```python
from build123d import *

# Parameters (mm, degrees)
SKETCH1_W           = 30
SKETCH1_H           = 90
BOSS_EXTRUDE1_DEPTH = 8
SKETCH2_W           = 10
SKETCH2_H           = 12
CUT_EXTRUDE1_DEPTH  = 8
SKETCH3_R           = 2.25
CUT_EXTRUDE2_DEPTH  = 55.671747731
FILLET1_R           = 2
CUT_EXTRUDE3_DEPTH  = 49.104053883
FILLET2_R           = 3
CHAMFER1_SIZE       = 1.5
FILLET3_R           = 0.5


with BuildPart() as part:
    # Sketch1 → Boss-Extrude1 (new body)
    with BuildSketch(Plane(origin=(0, 0, 0), x_dir=(1, 0, 0), z_dir=(0, 1, 0))):
        Rectangle(SKETCH1_W, SKETCH1_H)
    extrude(amount=BOSS_EXTRUDE1_DEPTH)

    # Sketch2 → Cut-Extrude1 (cut)
    with BuildSketch(Plane(origin=(0, 8, 0), x_dir=(1, 0, 0), z_dir=(0, 1, 0))):
        with Locations((0, 39)):
            Rectangle(SKETCH2_W, SKETCH2_H)
        with Locations((0, -39)):
            Rectangle(SKETCH2_W, SKETCH2_H)
    extrude(amount=-CUT_EXTRUDE1_DEPTH, mode=Mode.SUBTRACT)

    # Sketch3 → Cut-Extrude2 (cut, through all)
    with BuildSketch(Plane(origin=(15, 0, 0), x_dir=(0, 0, -1), z_dir=(1, 0, 0))):
        with Locations((-40, 4)):
            Circle(SKETCH3_R)
    cut_extrude2 = extrude(amount=-CUT_EXTRUDE2_DEPTH, mode=Mode.SUBTRACT)

    # Mirror1: Cut-Extrude2 across plane
    add(cut_extrude2.mirror(Plane.XY), mode=Mode.SUBTRACT)

    # Fillet1
    fillet1_edges = [part.edges().sort_by_distance(p)[0] for p in [
        (10, 0, 45),
        (-10, 0, -45),
        (-10, 8, 45),
        (-10, 8, -45),
        (10, 8, 45),
        (-10, 0, 45),
        (10, 0, -45),
        (10, 8, -45),
    ]]
    fillet(fillet1_edges, radius=FILLET1_R)

    # Sketch4 → Cut-Extrude3 (cut, through all)
    with BuildSketch(Plane(origin=(0, 8, 0), x_dir=(1, 0, 0), z_dir=(0, 1, 0))):
        Polygon((5, 26), (-10, 26), (1.641791045, 14.358208955), align=None)
        Polygon((10, 6), (10, 26), (5.52238806, 10.47761194), align=None)
        Polygon((-10, -6), (-10, -26), (-5.52238806, -10.47761194), align=None)
        Polygon((-5, -26), (10, -26), (-1.641791045, -14.358208955), align=None)
        Polygon((-10, 18.928932188), (-10, 1.071067812), (-3.939313176, -4.989619012), (0.058716162, 8.870216027), align=None)
        Polygon((9.840778775, -18.769710963), (9.840778775, -0.911846587), (3.939313176, 4.989619012), (-0.058716162, -8.870216027), align=None)
    extrude(amount=-CUT_EXTRUDE3_DEPTH, mode=Mode.SUBTRACT)

    # Fillet2
    fillet2_edges = [part.edges().sort_by_distance(p)[0] for p in [
        (0, 0, -33),
        (0, 0, 33),
    ]]
    fillet(fillet2_edges, radius=FILLET2_R)

    # Chamfer1
    chamfer1_edges = [part.edges().sort_by_distance(p)[0] for p in [
        (15, 4, -45),
        (15, 0, 0),
        (-15, 0, 0),
        (15, 8, 0),
        (15, 4, 45),
        (15, 7.414213562, 44.414213562),
        (15, 0.585786438, 44.414213562),
        (15, 7.414213562, -44.414213562),
        (15, 0.585786438, -44.414213562),
        (-15, 8, 0),
        (-15, 4, 45),
        (-15, 4, -45),
        (-15, 0.585786438, 44.414213562),
        (-15, 7.414213562, 44.414213562),
        (-15, 0.585786438, -44.414213562),
        (-15, 7.414213562, -44.414213562),
    ]]
    chamfer(chamfer1_edges, length=CHAMFER1_SIZE)

    # Fillet3
    fillet3_edges = [part.edges().sort_by_distance(p)[0] for p in [
        (-10, 4, -18.928932188),
        (0.058716162, 4, -8.870216027),
        (-3.939313176, 4, 4.989619012),
        (-10, 4, -1.071067812),
        (-1.641791045, 4, 14.358208955),
        (10, 4, 26),
        (-5, 4, 26),
        (10, 4, -6),
        (5.52238806, 4, -10.47761194),
        (10, 4, -26),
        (-10, 4, 6),
        (-5.52238806, 4, 10.47761194),
        (-10, 4, 26),
        (9.840778775, 4, 18.769710963),
        (-0.058716162, 4, 8.870216027),
        (3.939313176, 4, -4.989619012),
        (9.840778775, 4, 0.911846587),
        (5, 4, -26),
        (1.641791045, 4, -14.358208955),
        (-10, 4, -26),
    ]]
    fillet(fillet3_edges, radius=FILLET3_R)


solid = part.part
```
Model file for the job. Use its own axes, mm. A direction names the side the tool comes from. Coordinates: 2 decimals unless noted, no trailing zeros. Order: outer loops, then holes, each group sorted by start corner. A loop starts at its lowest first (then second) coordinate and runs counter-clockwise, first axis right, second up. Notation, with made-up numbers: (83, -39) -> (99, -39) arc R14 cw to (99, -16) -> close; hole circle Ø5 at (23, -26). An arc over 180 degrees is marked (long way). Answer as a JSON object with one key per item and string values. Group by question number.
1) Cut at A-A, the plane z = -40. Write the cut outline in (x, y).
2) Cut at D-D, the plane y = 4. Count the separate pieces of the cut face and the enclosed holes in it, then the cut area to 3 significant figures.
3) Flat gauge pins, fed straight in: pin 1 (4 mm diameter, centred on x = 2, y = 5.5, fed in from +Z); pin 2 (1.5 mm diameter, centred on y = 7, z = -1, fed in from +X); pin 3 (1.5 mm diameter, centred on x = 1, y = 5, fed in from -Z). Where does each tip first touch, or does it go through?
4) Which spindle directions (+Z, -Z, +X, -X, +Y, -Y) get a long thin tool onto all of the face, cutting with end or side? Do faces 1 (the face through (0, 0, -1)), 2 (the face through (4, 4, 20)). Say none if no direction does.
5) Cut at B-B, the plane z = 34. Write the cut outline in (x, y), then the cut area to 4 significant figures.
6) Drill centre lines: L1, parallel to Z at x = -11.5, y = 3.75; L2, parallel to X at y = 4, z = -3; L3, parallel to X at y = 4.25, z = -34.5. Where is each one in solid material? Low to high.
7) Cut at C-C, the plane z = 12. Write the cut outline in (x, y).
8) Pull direction X, two halves, no side cores. Call faces 3 (the face through (-9.93, 4.099, -42.248)), 4 (the face through (4.51, 4.06, 13.44)), 5 (the face through (15, 4, 1)), 6 (the face through (-14.3, 4, 44.2)): +X half, -X half, draft (parallel to the pull), parting line (faces both ways), or undercut.
Check values:
{
 "1": {"outline": "(-15, 1.5) -> (-13.5, 0) -> (-5, 0) -> (-5, 1.75) -> (-15, 1.75) -> close; (-15, 6.25) -> (-5, 6.25) -> (-5, 8) -> (-13.5, 8) -> (-15, 6.5) -> close; (5, 0) -> (13.5, 0) -> (15, 1.5) -> (15, 1.75) -> (5, 1.75) -> close; (5, 6.25) -> (15, 6.25) -> (15, 6.5) -> (13.5, 8) -> (5, 8) -> close"},
 "2": {"separate pieces": "5", "enclosed holes": "6", "area": "1,730 mm²"},
 "3": {"pin 1": "stops at z = 33", "pin 2": "stops at x = 15", "pin 3": "stops at z = -33"},
 "4": {"face 1": "+Z, -Z, +X, -X, -Y", "face 2": "+Y, -Y"},
 "5": {"outline": "(-15, 1.5) -> (-13.5, 0) -> (-5, 0) -> (-5, 8) -> (-13.5, 8) -> (-15, 6.5) -> close; (5, 0) -> (13.5, 0) -> (15, 1.5) -> (15, 6.5) -> (13.5, 8) -> (5, 8) -> close", "area": "155.5 mm²"},
 "6": {"L1": "z = -45 to -42.24, -37.76 to 37.76, 42.24 to 45", "L2": "x = -15 to -10, -1.63 to 3.37, 5.93 to 15", "L3": "x = -15 to -5, 5 to 15"},
 "7": {"outline": "(-15, 1.5) -> (-13.5, 0) -> (-10, 0) -> (-10, 8) -> (-13.5, 8) -> (-15, 6.5) -> close; (-5.96, 0) -> (3.07, 0) -> (3.07, 8) -> (-5.96, 8) -> close; (9.84, 0) -> (13.5, 0) -> (15, 1.5) -> (15, 6.5) -> (13.5, 8) -> (9.84, 8) -> close"},
 "8": {"face 3": "draft", "face 4": "undercut", "face 5": "+X half", "face 6": "-X half"}
}
